Read the model definition and answer for the solid it produces. Units are mm, in the model's axes. Coordinates: 2 decimals unless noted, no trailing zeros. Order: outer loops, then holes, each group sorted by start corner. A loop starts at its lowest first (then second) coordinate and runs counter-clockwise, first axis right, second up. Notation, with made-up numbers: M -27.5,1.5 L -6.5,1.5 A12 ccw -6.5,12.5 Z; hole C 32.25,25 d4. An arc over 180 degrees is marked long. One line per question, with ' | ' between items. Start each with the question number.
1) Find section B-B, the plane z = 0. Write down the section's boundary in (x, y).
2) Find section C-C, the plane x = 18. Write down the section's boundary in (y, z).
3) Consider probe 1 along X at (y, z) = (14, 0); probe 2 along Y at (x, z) = (46, 0); probe 3 along X at (y, z) = (25.5, -3). Determine where each line is inside the solid, lowest interval first.
4) Find section D-D, the plane z = 14. Write down the section's boundary in (x, y), plus the area to 3 significant figures.
5) Given P1, Ø11.5, axis at x = 49.5, z = 4, coming from the +Y side; P2, Ø5, axis at x = 13, y = 4.5, coming from the +Z side; P3, Ø6, axis at y = 29.5, z = 13.5, coming from the -X side, each flat-ended and moving along its own axis, determine where each tip first touches the part or whether it passes through.
6) Find section A-A, the plane y = 16. Write down the section's boundary in (x, z), plus the area to 3 significant figures.
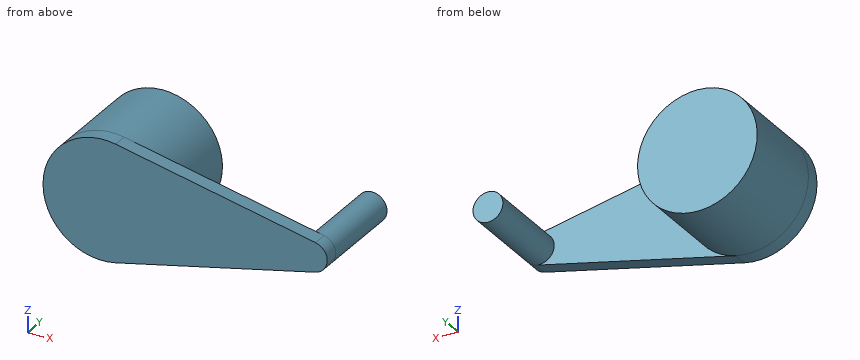
from build123d import *

# Parameters (mm, degrees)
EXTRUDE_1_DEPTH = 5
SKETCH_2_R      = 20
SKETCH_2_R_2    = 5
EXTRUDE_2_DEPTH = 30


with BuildPart() as part:
    # 草图1 → 凸台-拉伸1 (new body)
    with BuildSketch(Plane(origin=(0, 0, 0), x_dir=(1, 0, 0), z_dir=(0, 1, 0))):
        with BuildLine():
            Line((71.071428571, 4.883855118), (4.285714272, 19.535420476))
            ThreePointArc((4.285714272, 19.535420476), (-20, 1.6e-07), (4.28571396, -19.535420545))
            Line((4.28571396, -19.535420545), (71.071428571, -4.883855118))
            ThreePointArc((71.071428571, -4.883855118), (75, 0), (71.071428571, 4.883855118))
        make_face()
    extrude(amount=EXTRUDE_1_DEPTH)

    # 草图2 → 凸台-拉伸2 (add)
    with BuildSketch(Plane(origin=(0, 5, 0), x_dir=(1, 0, 0), z_dir=(0, 1, 0))):
        with Locations(Location((0, 0, 0), (0, 0, 77.626374884))):
            Circle(SKETCH_2_R)
        with Locations(Location((70, 0, 0), (0, 0, 77.626374884))):
            Circle(SKETCH_2_R_2)
    extrude(amount=EXTRUDE_2_DEPTH)


solid = part.part
Report:
1) outline: M -20,0 L 75,0 L 75,35 L 65,35 L 65,5 L 20,5 L 20,35 L -20,35 Z
2) outline: M 0,-16.53 L 5,-16.53 L 5,-8.72 L 35,-8.72 L 35,8.72 L 5,8.72 L 5,16.53 L 0,16.53 Z
3) probe 1: x = -20 to 20, 65 to 75 | probe 2: y = 0 to 5 | probe 3: x = -19.77 to 19.77, 66 to 74
4) outline: M -14.28,0 L 29.52,0 L 29.52,5 L 14.28,5 L 14.28,35 L -14.28,35 Z | area: 1,080 mm^2
5) P1: stops at y = 5 | P2: stops at z = 18.17 | P3: stops at x = -17.02
6) outline: C 0,0 d40; C 70,0 d10 | area: 1,340 mm^2
